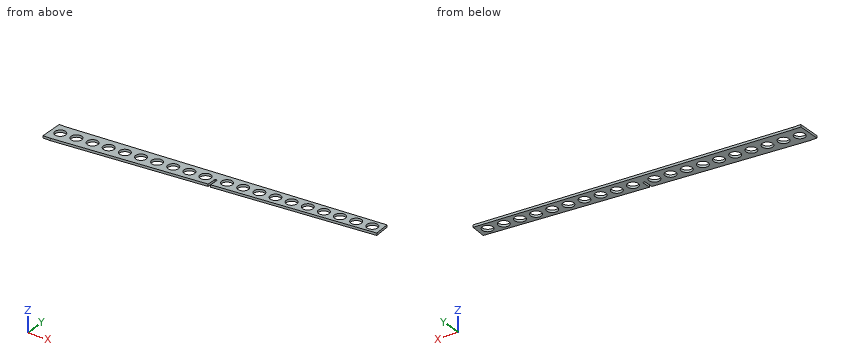
from build123d import *

# Parameters (mm, degrees)
BOSS_EXTRUDE1_DEPTH     = 3
SKETCH2_R               = 7
SKETCH2_W               = 3
SKETCH2_H               = 12.946630698
CUT_EXTRUDE1_DEPTH      = 1
CUT_EXTRUDE1_DEPTH_BACK = 4


with BuildPart() as part:
    # Sketch1 → Boss-Extrude1 (new body)
    with BuildSketch(Plane.XY):
        Polygon((-415, 0), (-415, 30), (-405, 30), (-0.732442974, 54.494049484), (0.732442974, 33.545204429), (-405, 0), align=None)
    extrude(amount=BOSS_EXTRUDE1_DEPTH)

    # Sketch2 → Cut-Extrude1 (cut, two sides)
    with BuildSketch(Plane.XY.offset(3)) as cut_extrude1_sk:
        with Locations((-403, 15.1433068)):
            Circle(SKETCH2_R)
        with Locations((-382.777777778, 16.592297775)):
            Circle(SKETCH2_R)
        with Locations((-362.555555556, 18.041288751)):
            Circle(SKETCH2_R)
        with Locations((-342.333333333, 19.490279727)):
            Circle(SKETCH2_R)
        with Locations((-322.111111111, 20.939270702)):
            Circle(SKETCH2_R)
        with Locations((-301.888888889, 22.388261678)):
            Circle(SKETCH2_R)
        with Locations((-281.666666667, 23.837252653)):
            Circle(SKETCH2_R)
        with Locations((-261.444444444, 25.286243629)):
            Circle(SKETCH2_R)
        with Locations((-241.222222222, 26.735234605)):
            Circle(SKETCH2_R)
        with Locations((-221, 28.18422558)):
            Circle(SKETCH2_R)
        with Locations((-194, 30.118867377)):
            Circle(SKETCH2_R)
        with Locations((-173.777777778, 31.567858353)):
            Circle(SKETCH2_R)
        with Locations((-153.555555556, 33.016849329)):
            Circle(SKETCH2_R)
        with Locations((-133.333333333, 34.465840304)):
            Circle(SKETCH2_R)
        with Locations((-113.111111111, 35.91483128)):
            Circle(SKETCH2_R)
        with Locations((-92.888888889, 37.363822255)):
            Circle(SKETCH2_R)
        with Locations((-72.666666667, 38.812813231)):
            Circle(SKETCH2_R)
        with Locations((-52.444444444, 40.261804207)):
            Circle(SKETCH2_R)
        with Locations((-32.222222222, 41.710795182)):
            Circle(SKETCH2_R)
        with Locations((-12, 43.159786158)):
            Circle(SKETCH2_R)
        with Locations((-207.5, 22.67823113)):
            Rectangle(SKETCH2_W, SKETCH2_H)
    extrude(amount=CUT_EXTRUDE1_DEPTH, mode=Mode.SUBTRACT)
    extrude(cut_extrude1_sk.sketch, amount=-CUT_EXTRUDE1_DEPTH_BACK, mode=Mode.SUBTRACT)


solid = part.part
Here's how the part is built. I have some questions about the finished solid (model axes, mm). Coordinates: 2 decimals unless noted, no trailing zeros. Order: outer loops, then holes, each group sorted by start corner. A loop starts at its lowest first (then second) coordinate and runs counter-clockwise, first axis right, second up. Notation, with made-up numbers: (-3, 36) -> (1, 36) arc R32 ccw to (1, 68) -> close; hole circle Ø10 at (39, 22). An arc over 180 degrees is marked (long way). Answer in a Markdown table with one row per item.
(1) Please list where these lines run through material, in increasing order: probe 1 along Y at (x, z) = (-71.5, 1.1); probe 2 along Y at (x, z) = (-78, 0.7); probe 3 along Y at (x, z) = (-312, 2.4).
Answer key:
| item | result |
|---|---|
| probe 1 | 27.57 to 31.91, 45.71 to 50.21 |
| probe 2 | 27.04 to 34.28, 43.35 to 49.81 |
| probe 3 | 7.69 to 35.63 |
(2) Will these pins go through, and if not, where does the flat tip stop? pin 1 Ø16 at (x, y) = (-52.44, 40.26) entering from +Z; pin 2 Ø1 at (y, z) = (45.5, 1) entering from +X; pin 3 Ø12.5 at (x, y) = (-261.44, 25.29) entering from +Z; pin 4 Ø1.5 at (x, z) = (-410.5, 2) entering from +Y.
Answer key:
| item | result |
|---|---|
| pin 1 | z = 3 |
| pin 2 | x = -0.07 |
| pin 3 | through |
| pin 4 | y = 30 |
(3) I want a section at B-B on z = 0.85. Count the separate pieces of the cut face and the enclosed holes in it, then the cut area to 3 significant figures.
Answer key:
| item | result |
|---|---|
| separate pieces | 1 |
| enclosed holes | 20 |
| area | 7,520 mm^2 |
(4) I want a section at A-A on x = -364. List the corners of the cut face in (y, z) for me.
Answer key:
| item | result |
|---|---|
| outline | (3.39, 0) -> (11.19, 0) -> (11.19, 3) -> (3.39, 3) -> close; (24.89, 0) -> (32.48, 0) -> (32.48, 3) -> (24.89, 3) -> close |
(5) I want a section at C-C on x = -12. List the corners of the cut face in (y, z) for me, then the cut area to 3 significant figures.
Answer key:
| item | result |
|---|---|
| outline | (32.49, 0) -> (36.16, 0) -> (36.16, 3) -> (32.49, 3) -> close; (50.16, 0) -> (53.81, 0) -> (53.81, 3) -> (50.16, 3) -> close |
| area | 22.0 mm^2 |
(6) I want a section at D-D on y = 4. List the corners of the cut face in (x, z) for me, then the cut area to 3 significant figures.
Answer key:
| item | result |
|---|---|
| outline | (-415, 0) -> (-356.62, 0) -> (-356.62, 3) -> (-415, 3) -> close |
| area | 175 mm^2 |
